CAD build for the part. Positions are in the model's coordinates, mm. A direction names the side the tool comes from. Give positions to 0.01 mm unless a question says otherwise; leave off trailing zeros. Loops run counter-clockwise (first coordinate to the right, second up) from the corner with the lowest first, then second, coordinate; pieces in that order, holes last. Notation, with made-up numbers: (28.25, 31) - (36.25, 31) arc R25 ccw to (36.25, 57) - close; hole circle Ø2 at (-12, 27). An arc over 180 degrees is marked (long way). Return JSON: item names as keys, results as strings.
from build123d import *
from build123d.topology import SkipClean

# Parameters (mm, degrees)
CUT_EXTRUDE1_DEPTH      = 285.72070999490006
CUT_EXTRUDE1_DEPTH_BACK = 285.72070999490006
SKETCH13_R              = 49.530000000000044
BOSS_EXTRUDE4_DEPTH     = 49.53


with BuildPart() as part:
    # Sketch1 → Revolve1 (revolve)
    with BuildSketch(Plane.XY, mode=Mode.PRIVATE) as revolve1_sk:
        with BuildLine():
            Line((-57.35114817524302, 46.95352330159362), (8.000000000000007, 49.53))
            Line((8.000000000000007, 49.53), (226.43999999999997, 49.529999999999994))
            ThreePointArc((226.43999999999997, 49.529999999999994), (261.4629988721697, 35.022998872169694), (275.96999999999997, 0))
            Line((275.96999999999997, 0), (-102.49, 0))
            ThreePointArc((-102.49, 0), (-89.37510555522056, 32.56589202866499), (-57.35114817524302, 46.95352330159362))
        make_face()
    revolve(revolve1_sk.sketch.rotate(Axis((-1000, 0, 0), (1, 0, 0)), 90), axis=Axis((-1000, 0, 0), (1, 0, 0)))

    # Sketch2 → Cut-Extrude1 (cut, two sides: drawn at the far end of the back side and taken through both)
    with BuildSketch(Plane(origin=(0, 0, 0), x_dir=(1, 0, 0), z_dir=(0, 1, 0)).offset(-CUT_EXTRUDE1_DEPTH_BACK)):
        Polygon((-102.49, 88.9), (-8.50999999999999, 88.9), (-8.50999999999998, 12.700000000000003), (-102.48999999999998, 12.7), align=None)
        Polygon((-102.48999999999998, -12.7), (-8.50999999999998, -12.700000000000003), (-8.50999999999999, -88.9), (-102.49, -88.9), align=None)
    extrude(amount=CUT_EXTRUDE1_DEPTH + CUT_EXTRUDE1_DEPTH_BACK, mode=Mode.SUBTRACT)

    # Sketch13 → Boss-Extrude4 (add)
    with SkipClean():  # the faces are left unmerged after this step: merging them gives an invalid solid
        with BuildSketch(Plane.XY):
            with Locations((226.43999999999997, 0)):
                Circle(SKETCH13_R)
        extrude(amount=BOSS_EXTRUDE4_DEPTH)

    # Sketch14 → Revolve4 (revolve)
    with SkipClean():  # the faces are left unmerged after this step: merging them gives an invalid solid
        with BuildSketch(Plane.XY.offset(49.53)):
            with BuildLine():
                Line((176.90999999999997, 0), (275.96999999999997, 1.82e-14))
                ThreePointArc((275.96999999999997, 1.82e-14), (226.43999999999997, 49.53), (176.90999999999997, 0))
            make_face()
        revolve(axis=Axis((176.90999999999997, 0, 49.53), (1, 1.8e-16, 0)))


solid = part.part
1. Which spindle directions (+Z, -Z, +X, -X, +Y, -Y) get a long thin tool onto all of the face, cutting with end or side? Do faces 1 (the face through (-8.51, -1, 27)), 2 (the face through (118.75, -2.18, -49.48)). Say none if no direction does.
Values follow:
{"face 1": "+Z, -X, +Y, -Y", "face 2": "-X"}
2. Drop flat-ended pins along their axis: P1, Ø8, axis at y = 17, z = 58, coming from the +X side; P2, Ø12, axis at x = 87, z = 51.5, coming from the +Y side; P3, Ø10, axis at x = 147, z = -16, coming from the +Y side. Give the stop position or say it passes through.
Values follow:
{"P1": "stops at x = 273.65", "P2": "stops at y = 19.57", "P3": "stops at y = 48.29"}
3. Cut at B-B, the plane z = 61. Write the cut outline in (x, y).
Values follow:
{"outline": "circle Ø96.37 at (226.44, 0)"}
4. Pull direction Z, two halves, no side cores. Call faces 3 (the face through (-8.51, -1, -27)), 4 (the face through (-55, -1, 12.7)), 5 (the face through (-54, -1, -12.7)): +Z half, -Z half, draft (parallel to the pull), parting line (faces both ways), or undercut.
Values follow:
{"face 3": "draft", "face 4": "+Z half", "face 5": "-Z half"}
5. Drill centre lines: probe 1 along Y at (x, z) = (-42.5, -7); probe 2 along Z at (x, y) = (-38, -33.5); probe 3 along Y at (x, z) = (-54, 0). Where is each one in solid material? Low to high.
Values follow:
{"probe 1": "y = -47.02 to 47.02", "probe 2": "z = -12.7 to 12.7", "probe 3": "y = -47.09 to 47.09"}
6. Cut at A-A, the plane x = 90. Write the cut outline in (y, z), plus the area to 3 significant figures.
Values follow:
{"outline": "circle Ø99.06 at (0, 0)", "area": "7,710 mm²"}
